Verification items for this drawing (mm, ordinates from the low corner). Give positions to 0.01 mm unless a question says otherwise; leave off trailing zeros. Loops run counter-clockwise (first coordinate to the right, second up) from the corner with the lowest first, then second, coordinate; pieces in that order, holes last. Notation, with made-up numbers: M 28.25,71.5 L 52.25,71.5 A17 cw 52.25,104.5 Z; hole C 76.25,63 d2. An arc over 180 degrees is marked long. Write each question's results on one line, items separated by ' | '. Start each with the question number.
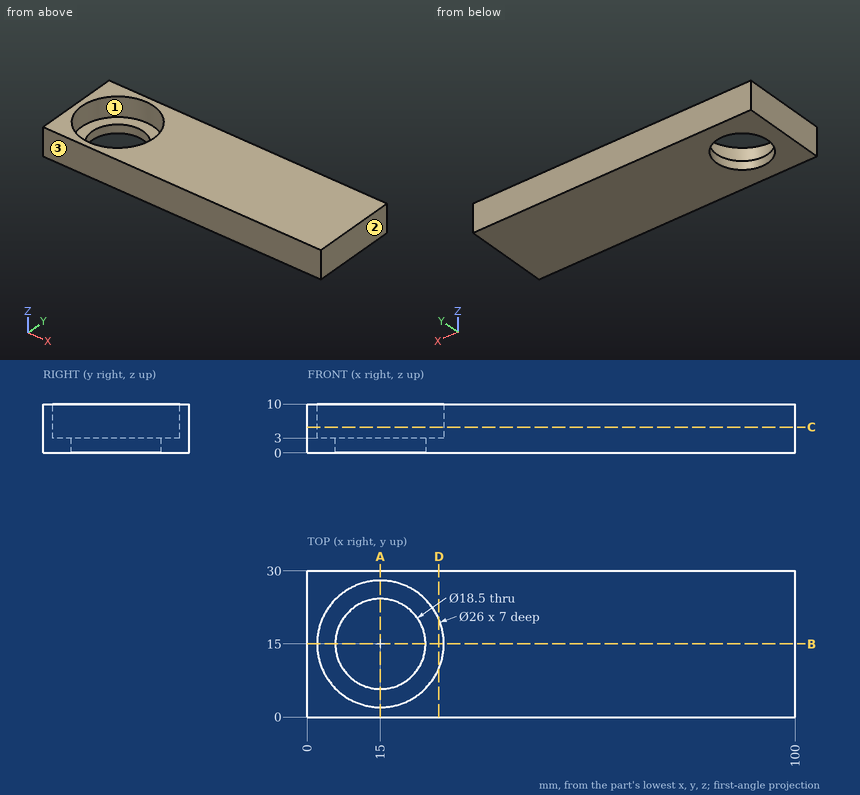
1. Section check A-A, the plane x = 15. Record the boundary of the cut face in (y, z), plus the area to 3 significant figures.
2. Section check D-D, the plane x = 27. Record the boundary of the cut face in (y, z), plus the area to 3 significant figures.
3. Section check C-C, the plane z = 5.25. Record the boundary of the cut face in (x, y), plus the area to 3 significant figures.
4. Thickness scan on probe 1 along Y at (x, z) = (15, 8); probe 2 along Y at (x, z) = (15, 1.25); probe 3 along X at (y, z) = (15.75, 5.25). Record the ranges inside material, lowest first.
5. Section check B-B, the plane y = 15. Record the boundary of the cut face in (x, z), plus the area to 4 significant figures.
6. Release check for a two-part mould opening along Y. For the marked faces 1, 2 and 3 record: released by +Y, released by -Y, zero draft, split by the parting line, or undercut.
Filled sheet:
1) outline: M 0,0 L 5.75,0 L 5.75,3 L 2,3 L 2,10 L 0,10 Z; M 24.25,0 L 30,0 L 30,10 L 28,10 L 28,3 L 24.25,3 Z | area: 62.5 mm2
2) outline: M 0,0 L 30,0 L 30,10 L 20,10 L 20,3 L 10,3 L 10,10 L 0,10 Z | area: 230 mm2
3) outline: M 0,0 L 100,0 L 100,30 L 0,30 Z; hole C 15,15 d26 | area: 2,470 mm2
4) probe 1: 0 to 2, 28 to 30 | probe 2: 0 to 5.75, 24.25 to 30 | probe 3: 0 to 2.02, 27.98 to 100
5) outline: M 0,0 L 5.75,0 L 5.75,3 L 2,3 L 2,10 L 0,10 Z; M 24.25,0 L 100,0 L 100,10 L 28,10 L 28,3 L 24.25,3 Z | area: 762.5 mm2
6) face 1: undercut | face 2: zero draft | face 3: released by -Y
